The listing builds one solid part. Answer for the finished solid, in the listing's coordinates (mm). A direction names the side the tool comes from. Coordinates: 2 decimals unless noted, no trailing zeros. Write each loop counter-clockwise with the first axis right and the second up, starting at its lowest first coordinate (ties: lowest second). Pieces come first, ordered by that corner, then holes.
```python
from build123d import *

# Parameters (mm, degrees)
CROQUIS1_W              = 22
CROQUIS1_H              = 35
CROQUIS1_R              = 1.6
SALIENTE_EXTRUIR1_DEPTH = 3
CROQUIS2_W              = 11.5
CROQUIS2_H              = 2.5
SALIENTE_EXTRUIR2_DEPTH = 9.9
CROQUIS4_R              = 2
CORTAR_EXTRUIR1_DEPTH   = 2.5
CORTAR_EXTRUIR2_START   = -2.5
CROQUIS5_R              = 2
CORTAR_EXTRUIR2_DEPTH   = 2.5
CROQUIS6_R              = 2.8
CORTAR_EXTRUIR3_DEPTH   = 0.3
REDONDEO1_R             = 2
REDONDEO2_R             = 10
REDONDEO4_R             = 2


# Some blends are built 0.0001 mm under size
with BuildPart() as part:
    # Croquis1 → Saliente-Extruir1 (new body)
    with BuildSketch(Plane(origin=(0, 0, 0), x_dir=(1, 0, 0), z_dir=(0, 1, 0))):
        with Locations((11, 17.5)):
            Rectangle(CROQUIS1_W, CROQUIS1_H)
        with Locations(Location((6, 27.5, 0), (0, 0, 270))):
            Circle(CROQUIS1_R, mode=Mode.SUBTRACT)
        with Locations(Location((6, 7.5, 0), (0, 0, 270))):
            Circle(CROQUIS1_R, mode=Mode.SUBTRACT)
    extrude(amount=SALIENTE_EXTRUIR1_DEPTH)

    # Croquis2 → Saliente-Extruir2 (add)
    with BuildSketch(Plane(origin=(0, 3, 0), x_dir=(1, 0, 0), z_dir=(0, 1, 0))):
        with Locations((16.25, 22.85)):
            Rectangle(CROQUIS2_W, CROQUIS2_H)
        with Locations((16.25, 12.15)):
            Rectangle(CROQUIS2_W, CROQUIS2_H)
    extrude(amount=SALIENTE_EXTRUIR2_DEPTH)

    # Croquis4 → Cortar-Extruir1 (cut)
    with BuildSketch(Plane.XY.offset(-21.6)):
        with Locations((16.25, 7)):
            Circle(CROQUIS4_R)
    extrude(amount=-CORTAR_EXTRUIR1_DEPTH, mode=Mode.SUBTRACT)

    # Croquis5 → Cortar-Extruir2 (cut)
    with BuildSketch(Plane(origin=(0, 0, -13.4), x_dir=(-1, 0, 0), z_dir=(0, 0, -1)).offset(CORTAR_EXTRUIR2_START)):
        with Locations(Location((-16.25, 7, 0), (0, 0, 180))):
            Circle(CROQUIS5_R)
    extrude(amount=CORTAR_EXTRUIR2_DEPTH, mode=Mode.SUBTRACT)

    # Croquis6 → Cortar-Extruir3 (cut)
    with BuildSketch(Plane(origin=(0, 3, 0), x_dir=(1, 0, 0), z_dir=(0, 1, 0))):
        with Locations(Location((6, 7.5, 0), (0, 0, 270))):
            Circle(CROQUIS6_R)
        with Locations(Location((6, 27.5, 0), (0, 0, 270))):
            Circle(CROQUIS6_R)
    extrude(amount=-CORTAR_EXTRUIR3_DEPTH, mode=Mode.SUBTRACT)

    # Redondeo1
    redondeo1_edges = [part.edges().sort_by_distance(p)[0] for p in [
        (14.25, 7, -21.6),
        (14.25, 7, -13.4),
    ]]
    fillet(redondeo1_edges, radius=REDONDEO1_R - 0.0001)  # a hair under: the kernel refuses the full size

    # Redondeo2
    # the kernel refuses this fillet: 10 mm, written as the material it adds along each edge
    with BuildSketch(Plane(origin=(22, 3, -24.1), x_dir=(0, 0, -1), z_dir=(-1, 0, 0))) as redondeo2_piece_1_section:
        with BuildLine():
            CenterArc((REDONDEO2_R, -REDONDEO2_R), REDONDEO2_R, 90, 90)
            Line((0, -REDONDEO2_R), (0, 0))
            Line((0, 0), (REDONDEO2_R, 0))
        make_face()
    redondeo2_piece_1 = extrude(amount=11.5, mode=Mode.PRIVATE)
    redondeo2_piece_1 = split(redondeo2_piece_1, bisect_by=Plane(origin=(12.416666667, 12.9, -31.511409781), z_dir=(0, -1, 0)), keep=Keep.TOP, mode=Mode.PRIVATE)
    redondeo2_piece_1 = redondeo2_piece_1 - Plane(origin=(16.25, 7, -31.511409781), x_dir=(1, 0, 0), z_dir=(0, 0, 1)) * Cylinder(2, 63, mode=Mode.PRIVATE)
    add(redondeo2_piece_1)
    with BuildSketch(Plane(origin=(10.5, 3, -24.1), x_dir=(-1, 0, 0), z_dir=(0, 0, 1))) as redondeo2_piece_2_section:
        with BuildLine():
            CenterArc((REDONDEO2_R, -REDONDEO2_R), REDONDEO2_R, 90, 90)
            Line((0, -REDONDEO2_R), (0, 0))
            Line((0, 0), (REDONDEO2_R, 0))
        make_face()
    redondeo2_piece_2 = extrude(amount=2.5, mode=Mode.PRIVATE)
    redondeo2_piece_2 = split(redondeo2_piece_2, bisect_by=Plane(origin=(8.234191854, 12.9, -22.85), z_dir=(0, -1, 0)), keep=Keep.TOP, mode=Mode.PRIVATE)
    add(redondeo2_piece_2)
    with BuildSketch(Plane(origin=(10.5, 3, -24.1), x_dir=(-1, 0, 0), z_dir=(0, 0, 1))) as redondeo2_piece_3_section:
        with BuildLine():
            CenterArc((REDONDEO2_R, -REDONDEO2_R), REDONDEO2_R, 90, 90)
            Line((0, -REDONDEO2_R), (0, 0))
            Line((0, 0), (REDONDEO2_R, 0))
        make_face()
    redondeo2_piece_3 = extrude(amount=27.5, mode=Mode.PRIVATE)
    redondeo2_piece_3 = split(redondeo2_piece_3, bisect_by=Plane(origin=(8.234191854, 5.257913166, -13.4), z_dir=(0, 0, 1)), keep=Keep.TOP, mode=Mode.PRIVATE)
    redondeo2_piece_3 = split(redondeo2_piece_3, bisect_by=Plane(origin=(8.234191854, 12.9, -12.15), z_dir=(0, -1, 0)), keep=Keep.TOP, mode=Mode.PRIVATE)
    redondeo2_piece_3 = split(redondeo2_piece_3, bisect_by=Plane(origin=(8.234191854, 5.257913166, -10.9), z_dir=(0, 0, -1)), keep=Keep.TOP, mode=Mode.PRIVATE)
    add(redondeo2_piece_3)
    with BuildSketch(Plane(origin=(10.5, 3, -38.4), x_dir=(-1, 0, 0), z_dir=(0, 0, 1))) as redondeo2_piece_4_section:
        with BuildLine():
            CenterArc((REDONDEO2_R, -REDONDEO2_R), REDONDEO2_R, 90, 90)
            Line((0, -REDONDEO2_R), (0, 0))
            Line((0, 0), (REDONDEO2_R, 0))
        make_face()
    redondeo2_piece_4 = extrude(amount=27.5, mode=Mode.PRIVATE)
    redondeo2_piece_4 = split(redondeo2_piece_4, bisect_by=Plane(origin=(8.234191854, 12.9, -22.85), z_dir=(0, -1, 0)), keep=Keep.TOP, mode=Mode.PRIVATE)
    redondeo2_piece_4 = split(redondeo2_piece_4, bisect_by=Plane(origin=(8.234191854, 5.257913166, -21.6), z_dir=(0, 0, -1)), keep=Keep.TOP, mode=Mode.PRIVATE)
    redondeo2_piece_4 = split(redondeo2_piece_4, bisect_by=Plane(origin=(8.234191854, 5.257913166, -24.1), z_dir=(0, 0, 1)), keep=Keep.TOP, mode=Mode.PRIVATE)
    add(redondeo2_piece_4)
    with BuildSketch(Plane(origin=(10.5, 3, -13.4), x_dir=(-1, 0, 0), z_dir=(0, 0, 1))) as redondeo2_piece_5_section:
        with BuildLine():
            CenterArc((REDONDEO2_R, -REDONDEO2_R), REDONDEO2_R, 90, 90)
            Line((0, -REDONDEO2_R), (0, 0))
            Line((0, 0), (REDONDEO2_R, 0))
        make_face()
    redondeo2_piece_5 = extrude(amount=2.5, mode=Mode.PRIVATE)
    redondeo2_piece_5 = split(redondeo2_piece_5, bisect_by=Plane(origin=(8.234191854, 12.9, -12.15), z_dir=(0, -1, 0)), keep=Keep.TOP, mode=Mode.PRIVATE)
    add(redondeo2_piece_5)
    with BuildSketch(Plane(origin=(10.5, 3, -10.9), x_dir=(0, 0, 1), z_dir=(1, 0, 0))) as redondeo2_piece_6_section:
        with BuildLine():
            CenterArc((REDONDEO2_R, -REDONDEO2_R), REDONDEO2_R, 90, 90)
            Line((0, -REDONDEO2_R), (0, 0))
            Line((0, 0), (REDONDEO2_R, 0))
        make_face()
    redondeo2_piece_6 = extrude(amount=11.5, mode=Mode.PRIVATE)
    redondeo2_piece_6 = split(redondeo2_piece_6, bisect_by=Plane(origin=(20.083333333, 12.9, -3.488590219), z_dir=(0, -1, 0)), keep=Keep.TOP, mode=Mode.PRIVATE)
    redondeo2_piece_6 = redondeo2_piece_6 - Plane(origin=(16.25, 7, -3.488590219), x_dir=(1, 0, 0), z_dir=(0, 0, 1)) * Cylinder(2, 63, mode=Mode.PRIVATE)
    add(redondeo2_piece_6)
    with BuildSketch(Plane(origin=(22, 3, -24.1), x_dir=(0, 0, -1), z_dir=(-1, 0, 0))) as redondeo2_piece_7a_section:
        with BuildLine():
            CenterArc((REDONDEO2_R, -REDONDEO2_R), REDONDEO2_R, 90, 90)
            Line((0, -REDONDEO2_R), (0, 0))
            Line((0, 0), (REDONDEO2_R, 0))
        make_face()
    redondeo2_piece_7a = extrude(amount=36.5, mode=Mode.PRIVATE)
    redondeo2_piece_7a = split(redondeo2_piece_7a, bisect_by=Plane(origin=(0, 3.280401031, -31.512996252), z_dir=(1, 0, 0)), keep=Keep.TOP, mode=Mode.PRIVATE)
    redondeo2_piece_7a = redondeo2_piece_7a - Plane(origin=(6, 3.280401031, -27.5), x_dir=(0, 0, 1), z_dir=(0, 1, 0)) * Cylinder(2.8, 113, mode=Mode.PRIVATE)
    redondeo2_piece_7a = split(redondeo2_piece_7a, bisect_by=Plane(origin=(1.75, 12.9, -31.512996252), z_dir=(0, -1, 0)), keep=Keep.TOP, mode=Mode.PRIVATE)
    redondeo2_piece_7a = split(redondeo2_piece_7a, bisect_by=Plane(origin=(10.5, 3.280401031, -31.512996252), z_dir=(-1, 0, 0)), keep=Keep.TOP, mode=Mode.PRIVATE)
    with BuildSketch(Plane(origin=(10.5, 3, -49.1), x_dir=(-1, 0, 0), z_dir=(0, 0, 1))) as redondeo2_piece_7b_section:
        with BuildLine():
            CenterArc((REDONDEO2_R, -REDONDEO2_R), REDONDEO2_R, 90, 90)
            Line((0, -REDONDEO2_R), (0, 0))
            Line((0, 0), (REDONDEO2_R, 0))
        make_face()
    redondeo2_piece_7b = extrude(amount=27.5, mode=Mode.PRIVATE)
    redondeo2_piece_7b = split(redondeo2_piece_7b, bisect_by=Plane(origin=(8.577465214, 5.522304582, -35), z_dir=(0, 0, 1)), keep=Keep.TOP, mode=Mode.PRIVATE)
    redondeo2_piece_7b = redondeo2_piece_7b - Plane(origin=(6, 5.522304582, -27.5), x_dir=(0, 0, 1), z_dir=(0, 1, 0)) * Cylinder(2.8, 95, mode=Mode.PRIVATE)
    redondeo2_piece_7b = split(redondeo2_piece_7b, bisect_by=Plane(origin=(8.577465214, 12.9, -29.998804987), z_dir=(0, -1, 0)), keep=Keep.TOP, mode=Mode.PRIVATE)
    redondeo2_piece_7b = split(redondeo2_piece_7b, bisect_by=Plane(origin=(8.577465214, 5.522304582, -24.1), z_dir=(0, 0, -1)), keep=Keep.TOP, mode=Mode.PRIVATE)
    redondeo2_piece_7 = redondeo2_piece_7a & redondeo2_piece_7b
    add(redondeo2_piece_7)
    with BuildSketch(Plane(origin=(-14.5, 3, -10.9), x_dir=(0, 0, 1), z_dir=(1, 0, 0))) as redondeo2_piece_8a_section:
        with BuildLine():
            CenterArc((REDONDEO2_R, -REDONDEO2_R), REDONDEO2_R, 90, 90)
            Line((0, -REDONDEO2_R), (0, 0))
            Line((0, 0), (REDONDEO2_R, 0))
        make_face()
    redondeo2_piece_8a = extrude(amount=36.5, mode=Mode.PRIVATE)
    redondeo2_piece_8a = split(redondeo2_piece_8a, bisect_by=Plane(origin=(0, 3.280397801, -3.487004608), z_dir=(1, 0, 0)), keep=Keep.TOP, mode=Mode.PRIVATE)
    redondeo2_piece_8a = redondeo2_piece_8a - Plane(origin=(6, 3.280397801, -7.5), x_dir=(0, 0, 1), z_dir=(0, 1, 0)) * Cylinder(2.8, 113, mode=Mode.PRIVATE)
    redondeo2_piece_8a = split(redondeo2_piece_8a, bisect_by=Plane(origin=(8.75, 12.9, -3.487004608), z_dir=(0, -1, 0)), keep=Keep.TOP, mode=Mode.PRIVATE)
    redondeo2_piece_8a = split(redondeo2_piece_8a, bisect_by=Plane(origin=(10.5, 3.280397801, -3.487004608), z_dir=(-1, 0, 0)), keep=Keep.TOP, mode=Mode.PRIVATE)
    with BuildSketch(Plane(origin=(10.5, 3, -13.4), x_dir=(-1, 0, 0), z_dir=(0, 0, 1))) as redondeo2_piece_8b_section:
        with BuildLine():
            CenterArc((REDONDEO2_R, -REDONDEO2_R), REDONDEO2_R, 90, 90)
            Line((0, -REDONDEO2_R), (0, 0))
            Line((0, 0), (REDONDEO2_R, 0))
        make_face()
    redondeo2_piece_8b = extrude(amount=27.5, mode=Mode.PRIVATE)
    redondeo2_piece_8b = split(redondeo2_piece_8b, bisect_by=Plane(origin=(8.577464667, 5.522304516, 0), z_dir=(0, 0, -1)), keep=Keep.TOP, mode=Mode.PRIVATE)
    redondeo2_piece_8b = redondeo2_piece_8b - Plane(origin=(6, 5.522304516, -7.5), x_dir=(0, 0, 1), z_dir=(0, 1, 0)) * Cylinder(2.8, 95, mode=Mode.PRIVATE)
    redondeo2_piece_8b = split(redondeo2_piece_8b, bisect_by=Plane(origin=(8.577464667, 12.9, -5.00119928), z_dir=(0, -1, 0)), keep=Keep.TOP, mode=Mode.PRIVATE)
    redondeo2_piece_8b = split(redondeo2_piece_8b, bisect_by=Plane(origin=(8.577464667, 5.522304516, -10.9), z_dir=(0, 0, 1)), keep=Keep.TOP, mode=Mode.PRIVATE)
    redondeo2_piece_8 = redondeo2_piece_8a & redondeo2_piece_8b
    add(redondeo2_piece_8)

    # Redondeo4
    redondeo4_edges = [part.edges().sort_by_distance(p)[0] for p in [
        (0, 1.5, -35),
        (0, 1.5, 0),
        (22, 1.5, 0),
        (22, 1.5, -35),
    ]]
    fillet(redondeo4_edges, radius=REDONDEO4_R)


solid = part.part
```
(1) For a pull along Z with two mould halves and no side action, classify faces 1 (the flat face through (11, 0, -18)), 2 (the cylindrical face through (8.36, 3.91, -25.99)), 3 (the flat face through (13, 10, -21.6)), 4 (the cylindrical face through (0.6, 1.52, -0.57)) as pulls with the +Z half, pulls with the -Z half, needs draft (parallel to the pull), parting line crosses it, or undercut.
(2) Find the intervals of material crossed by probe 1 along X at (y, z) = (1, -7.5); probe 2 along Y at (x, z) = (16.25, -11.3); probe 3 along Z at (x, y) = (10, 8.75), in increasing order.
(3) Which of the six approach directions +Z, -Z, +X, -X, +Y, -Y give full straight-line access (tool end or side, diameter ignored) to faces 5 (the flat face through (5, 2.7, -26)), 6 (the cylindrical face through (4.44, 1.33, -7.85))?
(4) Section D-D, the plane z = -7.5 is taken. Write down the section's boundary in (x, y).
(5) Each of these flat-tipped pins is pushed along its axis until it touches: pin 1 (6.5 mm diameter, centred on x = 16.25, y = 7, fed in from +Z); pin 2 (1.5 mm diameter, centred on x = 18, y = 5, fed in from -Z); pin 3 (9 mm diameter, centred on x = 6, z = -7.5, fed in from +Y). Where does it stop, or does it pass through?
(6) Section B-B, the plane z = -12.5 is taken. Write down the section's boundary in (x, y).
(7) Section A-A, the plane y = 2.25 is taken. Write down the section's boundary in (x, z).
(8) Section C-C, the plane x = 6 is taken. Write down the section's boundary in (y, z).
Solution:
1. face 1: needs draft
1. face 2: undercut
1. face 3: undercut
1. face 4: pulls with the +Z half
2. probe 1: x = 0 to 4.4, 7.6 to 22
2. probe 2: y = 0 to 5, 9 to 12.9
2. probe 3: z = -25.05 to -21.6, -13.4 to -9.95
3. face 5: +Y
3. face 6: +Y, -Y
4. outline: (0, 0) - (4.4, 0) - (4.4, 2.7) - (3.2, 2.7) - (3.2, 3.37) arc R10 cw to (0.5, 3) - (0, 3) - close; (7.6, 0) - (22, 0) - (22, 5.49) - (17.56, 5.49) arc R2 cw to (14.94, 5.49) - (8.8, 5.49) - (8.8, 2.7) - (7.6, 2.7) - close
5. pin 1: stops at z = -4.7
5. pin 2: stops at z = -29.26
5. pin 3: stops at y = 9.04
6. outline: (0, 0) - (22, 0) - (22, 12.9) - (10.5, 12.9) arc R10 cw to (0.5, 3) - (0, 3) - close; hole circle Ø4.66 at (16.25, 7)
7. outline: (0, -33) arc R2 ccw to (2, -35) - (20, -35) arc R2 ccw to (22, -33) - (22, -2) arc R2 ccw to (20, 0) - (2, 0) arc R2 ccw to (0, -2) - close; hole circle Ø3.2 at (6, -27.5); hole circle Ø3.2 at (6, -7.5)
8. outline: (0, -35) - (3, -35) - (3, -34.1) arc R10 cw to (3.75, -30.3) - (2.7, -30.3) - (2.7, -29.1) - (0, -29.1) - close; (0, -25.9) - (2.7, -25.9) - (2.7, -24.7) - (4.65, -24.7) - (4.65, -21.6) - (3, -21.6) - (3, -13.4) - (4.65, -13.4) - (4.65, -10.3) - (2.7, -10.3) - (2.7, -9.1) - (0, -9.1) - close; (0, -5.9) - (2.7, -5.9) - (2.7, -4.7) - (3.75, -4.7) arc R10 cw to (3, -0.9) - (3, 0) - (0, 0) - close
